Input: dimensioned drawing with shaded views. Units: mm. Origin: part minimum x, y, z. A direction names the side the tool comes from. Coordinates: 2 decimals unless noted, no trailing zeros. Loops run counter-clockwise (first coordinate to the right, second up) from the corner with the lowest first, then second, coordinate; pieces in that order, holes last. Notation, with made-up numbers: (70, -15) - (80, -15) arc R18 ccw to (80, 19) - close; hole circle Ø5 at (-3.5, 10). An arc over 180 degrees is marked (long way). Put each result on its own line as item: value. Start each with the question number.
1) Section D-D on z = 21.25. Output: boundary loops of the cut face in (x, y), and give its area (3 significant figures).
2) Material intervals for line 1 along X through (y, z) = (16.6, 9.75); line 2 along Y through (x, z) = (24.8, 7.75); line 3 along Y through (x, z) = (4.8, 4), sorted ascending. Write a range as from..to.
3) Section B-B on z = 7.75. Output: boundary loops of the cut face in (x, y).
4) Reachability of the marked faces 4 and 5 from +Z, -Z, +X, -X, +Y, -Y: full face, straight path, thin tool, end or side. Return the list, or none.
5) Section C-C on x = 14.8. Output: boundary loops of the cut face in (y, z), and give its area (3 significant figures).
6) Contact query for flat-ended pins moving along their axis: pin 1 Ø4 at (y, z) = (25, 13) entering from -X; pin 2 Ø1.5 at (x, y) = (24.5, 17) entering from -Z. Output: stop coordinate, or through.
7) Section A-A on y = 16.6. Output: boundary loops of the cut face in (x, z).
8) Draft query along X for the marked faces 1, 2 and 3. Return one class per face: +X half, -X half, draft (parallel to the pull), parting line (faces both ways), or undercut.
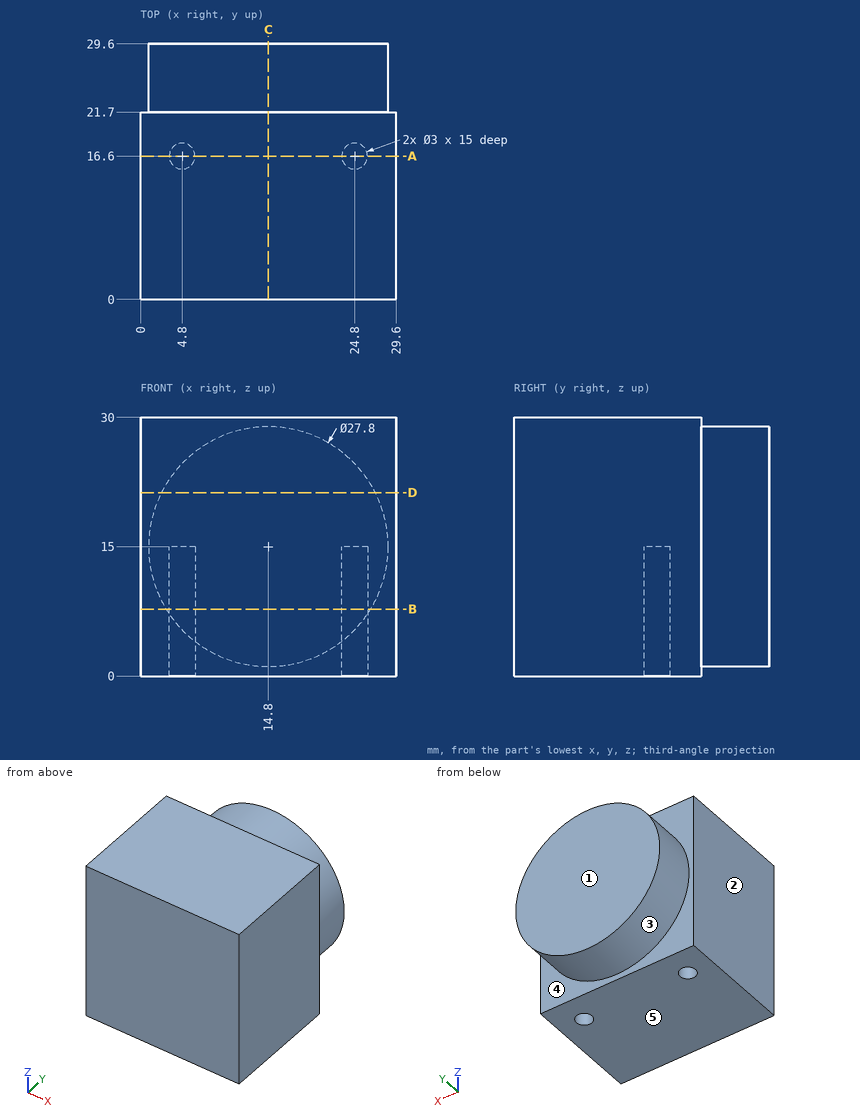
Answer block:
1. outline: (0, 0) - (29.6, 0) - (29.6, 21.7) - (27.22, 21.7) - (27.22, 29.6) - (2.38, 29.6) - (2.38, 21.7) - (0, 21.7) - close
1. area: 838 mm²
2. line 1: x = 0..3.3, 6.3..23.3, 26.3..29.6
2. line 2: y = 0..15.1, 18.1..29.6
2. line 3: y = 0..15.1, 18.1..21.7
3. outline: (0, 0) - (29.6, 0) - (29.6, 21.7) - (26.66, 21.7) - (26.66, 29.6) - (2.94, 29.6) - (2.94, 21.7) - (0, 21.7) - close; hole circle Ø3 at (4.8, 16.6); hole circle Ø3 at (24.8, 16.6)
4. face 4: +Y
4. face 5: -Z, +X, -X, +Y, -Y
5. outline: (0, 0) - (21.7, 0) - (21.7, 1.1) - (29.6, 1.1) - (29.6, 28.9) - (21.7, 28.9) - (21.7, 30) - (0, 30) - close
5. area: 871 mm²
6. pin 1: stops at x = 0.9
6. pin 2: stops at z = 15
7. outline: (0, 0) - (3.3, 0) - (3.3, 15) - (6.3, 15) - (6.3, 0) - (23.3, 0) - (23.3, 15) - (26.3, 15) - (26.3, 0) - (29.6, 0) - (29.6, 30) - (0, 30) - close
8. face 1: draft
8. face 2: -X half
8. face 3: parting line
